Geometry: final body of the model. Coordinates: model frame, mm. Face numbers are marked on the shaded views. Give positions to 0.01 mm unless a question says otherwise; leave off trailing zeros. Write each loop counter-clockwise with the first axis right and the second up, starting at its lowest first coordinate (ties: lowest second). Pieces come first, ordered by that corner, then holes.
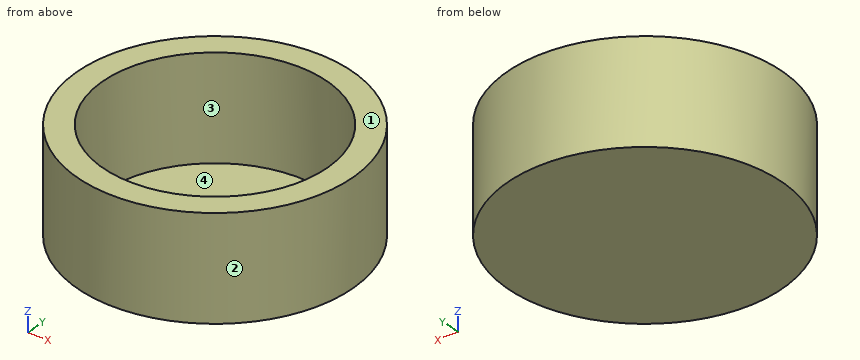
Autodesk Inventor part; units mm, degrees
ref_plane "YZ Plane" through (0, 0, 0) normal (1, 0, 0) x (0, 1, 0)
ref_plane "XZ Plane" through (0, 0, 0) normal (0, 1, 0) x (-1, 0, 0)
ref_plane "XY Plane" through (0, 0, 0) normal (0, 0, 1) x (1, 0, 0)
sketch "Sketch1" plane through (0, 0, 0) normal (0, 0, 1) x (1, 0, 0)
  circle A0 centre (0, 0) radius 42.5
  dimension "d0" = 85
extrude "Extrusion1" add sketch "Sketch1" along normal blind 31.93
sketch "Sketch2" plane through (0, 0, 31.93) normal (0, 0, 1) x (1, 0, 0)
  circle A0 centre (0, 0) radius 34.67
  circle A1 centre (0, 0) radius 42.5
  dimension "d3" = 7.83
extrude "Extrusion2" cut sketch "Sketch2" against normal blind 31.92 contours A0
sketch "Sketch5" plane through (0, 0, 0.01) normal (0, 0, 1) x (1, 0, 0)
  line L0 (3.2417, 5.6147) -> (6.4833, 0)
  line L1 (6.4833, 0) -> (3.2417, -5.6147)
  line L2 (3.2417, -5.6147) -> (-3.2417, -5.6147)
  line L3 (-3.2417, -5.6147) -> (-6.4833, 0)
  line L4 (-6.4833, 0) -> (-3.2417, 5.6147)
  line L5 (-3.2417, 5.6147) -> (3.2417, 5.6147)
  line L6 (-59.5, 0) -> (59.5, 0)
  line L7 (0, -59.5) -> (0, 59.5)
  circle A0 centre (0, 0) radius 6.4833
  circle A1 centre (0, 0) radius 8.1344
  dimension "d13" = 12.9667
  dimension "d14" = 1.651
extrude "Extrusion5" add sketch "Sketch5" along normal blind 3.0734 contours A0 L0 | A0 L7 A1 L6 | L5 L7 A0 | A0 L1 | L6 A1 L7 A0 | L5 A0 L7 | A0 L6 A1 L7 | A0 L7 L2 | L4 A0 | L7 A0 L2 | L7 A1 L6 A0 | L3 A0
properties part number "wheel"
Item 1: Section A-A, the plane x = 0. Return the cut outline in (y, z).
Found:
outline: (-42.5, 0) - (42.5, 0) - (42.5, 31.93) - (34.67, 31.93) - (34.67, 0.01) - (8.13, 0.01) - (8.13, 3.08) - (5.61, 3.08) - (5.61, 0.01) - (-5.61, 0.01) - (-5.61, 3.08) - (-8.13, 3.08) - (-8.13, 0.01) - (-34.67, 0.01) - (-34.67, 31.93) - (-42.5, 31.93) - close
Item 2: Section B-B, the plane z = 28. Return the cut outline in (x, y), plus the area to 3 significant figures.
Found:
outline: circle Ø85 at (0, 0); hole circle Ø69.34 at (0, 0)
area: 1,900 mm2
Item 3: Section C-C, the plane y = -19. Return the cut outline in (x, z), plus the area to 3 significant figures.
Found:
outline: (-38.02, 0) - (38.02, 0) - (38.02, 31.93) - (29, 31.93) - (29, 0.01) - (-29, 0.01) - (-29, 31.93) - (-38.02, 31.93) - close
area: 576 mm2
Item 4: Line query: L1, parallel to Y at x = 0, z = 10.5; L2, parallel to X at y = 13.5, z = 2; L3, parallel to Y at x = 24.5, z = 28. Output: solid intervals per line, ascending.
Found:
L1: y = -42.5 to -34.67, 34.67 to 42.5
L2: x = -40.3 to -31.93, 31.93 to 40.3
L3: y = -34.73 to -24.53, 24.53 to 34.73
Item 5: Pull-direction query (Y, two-part tool) for the marked faces 1, 2, 3 and 4; classes: +Y half, -Y half, draft (parallel to the pull), parting line (faces both ways), or undercut.
Found:
face 1: draft
face 2: parting line
face 3: undercut
face 4: undercut
Item 6: Section D-D, the plane x = -23. Return the cut outline in (y, z), plus the area to 3 significant figures.
Found:
outline: (-35.74, 0) - (35.74, 0) - (35.74, 31.93) - (25.94, 31.93) - (25.94, 0.01) - (-25.94, 0.01) - (-25.94, 31.93) - (-35.74, 31.93) - close
area: 626 mm2
Item 7: Pin query (flat end, axial travel): pin 1 Ø5.5 at (x, y) = (1, -1.5) entering from +Z; pin 2 Ø8 at (y, z) = (-5.5, 20.5) entering from -X; pin 3 Ø10 at (x, z) = (2.5, 22) entering from +Y. Return the tip coordinate at first contact, or that it passes through.
Found:
pin 1: stops at z = 0.01
pin 2: stops at x = -42.47
pin 3: stops at y = 42.5
